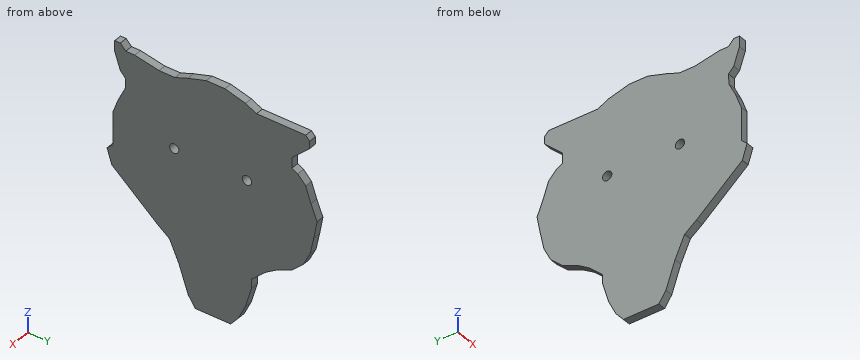
```python
from build123d import *

# Parameters (mm, degrees)
F1_DEPTH = 4.2
F3_D     = 5
F3_DEPTH = 12


with BuildPart() as f1:
    # F0 (on Right) → F1 (new body)
    with BuildSketch(Plane.YZ):
        Polygon((-46.670854, 44.319186), (-46.927813, 38.92304), (-50.525237, 31.728189), (-53.608745, 23.505505), (-53.608745, 17.595448), (-53.608745, 10.657554), (-53.608745, 6.032293), (-56.692254, 3.205744), (-54.122664, -4.759984), (-29.454602, -25.830621), (-23.030626, -30.712841), (-17.891448, -42.019036), (-13.009225, -56.151781), (-9.154841, -61.804876), (-3.244784, -61.804876), (3.693108, -61.804876), (9.860124, -61.804876), (13.97147, -56.922659), (17.825851, -48.956931), (21.166321, -37.650734), (21.166321, -33.025473), (28.361171, -26.344538), (34.01427, -22.747112), (42.750873, -18.892728), (49.009407, -13.081229), (52.679341, -5.741356), (54.570988, 3.205744), (56.369703, 12.713227), (53.029235, 20.935914), (50.202683, 29.158602), (45.956173, 33.731764), (42.754392, 35.332654), (42.754392, 38.409129), (42.754392, 40.978711), (46.921574, 44.84824), (52.35221, 49.890975), (52.35221, 53.826664), (50.202683, 56.141538), (42.754392, 56.141538), (32.215554, 56.141538), (23.735909, 56.141538), (17.825851, 59.096566), (6.776613, 62.049348), (3.693108, 62.049348), (-3.244784, 62.049348), (-13.266183, 58.965843), (-20.204078, 56.396253), (-28.683724, 56.396253), (-41.78863, 58.965843), (-46.670854, 58.965843), (-49.53411, 62.049348), (-52.580908, 62.049348), (-52.580908, 56.396253), (-49.53411, 47.402691), align=None)
    extrude(amount=F1_DEPTH)

    # F3
    with Locations(Plane.YZ.offset(4.2)):
        with Locations((-20.545784, 18.379813), (18.616695, 18.379813)):
            Hole(F3_D / 2, depth=F3_DEPTH)


solid = f1.part
```
The listing builds one solid part. Answer for the finished solid, in the listing's coordinates (mm). Give positions to 0.01 mm unless a question says otherwise; leave off trailing zeros. Order: outer loops, then holes, each group sorted by start corner. A loop starts at its lowest first (then second) coordinate and runs counter-clockwise, first axis right, second up. Notation, with made-up numbers: (-16, 86) -> (-3, 86) arc R37 cw to (-3, 125) -> close; hole circle Ø10 at (37.5, 80). An arc over 180 degrees is marked (long way). Answer as a JSON object with one key per item and string values. Group by question number.
Item 1: The part is cut by section C-C on x = 1.15. Give the number of separate pieces and of enclosed holes in the cut face, and give its area (3 significant figures).
Item 2: The part is cut by section A-A on z = -14.5. Write down the section's boundary in (x, y), and give its area (3 significant figures).
Item 3: The part is cut by section B-B on y = 41. Write down the section's boundary in (x, z).
Item 4: Consider L1, parallel to Z at x = 1.85, y = 34; L2, parallel to Y at x = 0.6, z = 19; L3, parallel to Y at x = 0.3, z = -37. Determine where each line is inside the solid, lowest interval first. Write a range as from..to.
Item 5: Flat-ended cylindrical pins translate along their axes: pin 1 (2 mm diameter, centred on x = 3, z = 13, fed in from -Y); pin 2 (1.3 mm diameter, centred on x = 1.5, y = -26.5, fed in from +Z); pin 3 (2 mm diameter, centred on x = 0.5, z = 6.5, fed in from +Y). Find the tip coordinate at first contact, or state that the pin passes through.
Result set:
{
 "1": {"separate pieces": "1", "enclosed holes": "2", "area": "9,610 mm²"},
 "2": {"outline": "(0, -42.72) -> (4.2, -42.72) -> (4.2, 47.48) -> (0, 47.48) -> close", "area": "379 mm²"},
 "3": {"outline": "(0, -19.67) -> (4.2, -19.67) -> (4.2, 56.14) -> (0, 56.14) -> close"},
 "4": {"L1": "-22.76..56.14", "L2": "-53.61..-22.97, -18.12..16.19, 21.04..53.82", "L3": "-20.17..21.17"},
 "5": {"pin 1": "y = -53.61", "pin 2": "z = 56.4", "pin 3": "y = 55.38"}
}
